Input: part model. Units: mm. Frame: model coordinates. Face numbers are marked on the shaded views. A direction names the side the tool comes from. Coordinates: 2 decimals unless noted, no trailing zeros. Order: outer loops, then holes, each group sorted by start corner. A loop starts at its lowest first (then second) coordinate and runs counter-clockwise, first axis right, second up. Notation, with made-up numbers: (59, 83.5) -> (90, 83.5) arc R14 ccw to (90, 109.5) -> close; hole circle Ø9 at (7, 33.5). An arc over 180 degrees is marked (long way). One line per item, written item: value. Start each with the question number.
from build123d import *

# Parameters (mm, degrees)
F1_DEPTH = 50.8
F3_DEPTH = 25.4
F4_DEPTH = 50.8


with BuildPart() as f1:
    # F0 (on Top) → F1 (new body)
    with BuildSketch(Plane.XY):
        with BuildLine():
            ThreePointArc((-15.1947466657, 0), (-22.0060110943, -10.86221038), (-25.7512666285, -23.1241025031))
            ThreePointArc((-25.7512666285, -23.1241025031), (-2.0484127491, -44.6133454073), (23.3222842216, -25.1212809235))
            ThreePointArc((23.3222842216, -25.1212809235), (21.5555211936, -11.7044416716), (14.7629464045, 0))
            ThreePointArc((14.7629464045, 0), (10.7387450248, 12.5467581674), (14.7629464045, 25.0935163349))
            ThreePointArc((14.7629464045, 25.0935163349), (21.5180813897, 36.4983696165), (23.3222842216, 49.63029176))
            Line((23.3222842216, 49.63029176), (-25.7512666285, 49.63029176))
            ThreePointArc((-25.7512666285, 49.63029176), (-22.2790381522, 36.5848904706), (-15.1947466657, 25.0935163349))
            ThreePointArc((-15.1947466657, 25.0935163349), (-10.9623069939, 12.5467581674), (-15.1947466657, 0))
        make_face()
    extrude(amount=F1_DEPTH)

    # F2 (on Right) → F3 (cut)
    with BuildSketch(Plane.YZ):
        with BuildLine():
            ThreePointArc((24.7435215861, 0), (0.6627701223, 5.5987162901), (-23.4179813415, 0))
            Line((-23.4179813415, 0), (24.7435215861, 0))
        make_face()
        with BuildLine():
            ThreePointArc((-46.2089851499, 24.0807514638), (-34.8134832457, 29.0446018263), (-23.4179813415, 24.0807514638))
            ThreePointArc((-23.4179813415, 24.0807514638), (0.6627701223, 14.6606816853), (24.7435215861, 24.0807514638))
            add(Edge.make_bspline(
                [(24.7435215861, 24.0807514638), (26.9770560839, 27.0474434767), (31.7641691677, 33.4059260361), (45.7356507893, 42.0064080333), (49.0760807653, 41.9577828011), (50.1966327429, 41.9414713979)],
                knots=[0, 0, 0, 0, 0.3675927898, 0.7878581036, 1, 1, 1, 1], degree=3))
            Line((50.1966327429, 41.9414713979), (50.1966327429, 52.80091241))
            Line((50.1966327429, 52.80091241), (-46.2089851499, 52.80091241))
            Line((-46.2089851499, 52.80091241), (-46.2089851499, 24.0807514638))
        make_face()
    extrude(amount=F3_DEPTH, mode=Mode.SUBTRACT)

    # F2 (on Right) → F4 (cut)
    with BuildSketch(Plane.YZ):
        with BuildLine():
            ThreePointArc((-46.2089851499, 24.0807514638), (-34.8134832457, 29.0446018263), (-23.4179813415, 24.0807514638))
            ThreePointArc((-23.4179813415, 24.0807514638), (0.6627701223, 14.6606816853), (24.7435215861, 24.0807514638))
            add(Edge.make_bspline(
                [(24.7435215861, 24.0807514638), (26.9770560839, 27.0474434767), (31.7641691677, 33.4059260361), (45.7356507893, 42.0064080333), (49.0760807653, 41.9577828011), (50.1966327429, 41.9414713979)],
                knots=[0, 0, 0, 0, 0.3675927898, 0.7878581036, 1, 1, 1, 1], degree=3))
            Line((50.1966327429, 41.9414713979), (50.1966327429, 52.80091241))
            Line((50.1966327429, 52.80091241), (-46.2089851499, 52.80091241))
            Line((-46.2089851499, 52.80091241), (-46.2089851499, 24.0807514638))
        make_face()
        with BuildLine():
            ThreePointArc((24.7435215861, 0), (0.6627701223, 5.5987162901), (-23.4179813415, 0))
            Line((-23.4179813415, 0), (24.7435215861, 0))
        make_face()
    extrude(amount=-F4_DEPTH, mode=Mode.SUBTRACT)


solid = f1.part
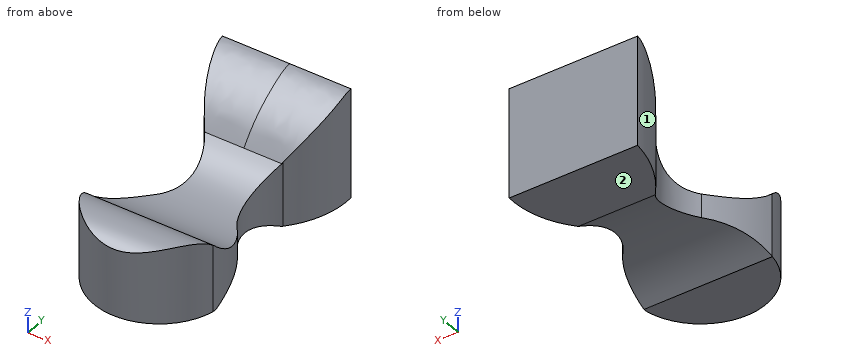
1) Section query A-A, the plane z = 9. Return the cut outline in (x, y), plus the area to 3 significant figures.
2) Ray query, line 1 along Y through (x, z) = (-16, 26); line 2 along Y through (x, z) = (17.5, 22); line 3 along X through (y, z) = (11, 8). Return the intervals inside material, ascending. Write a range as from..to.
3) Pin query (flat end, axial travel): pin 1 Ø8 at (x, y) = (11, 3) entering from +Z; pin 2 Ø12 at (y, z) = (-14, 18) entering from -X; pin 3 Ø10 at (y, z) = (-12, 7) entering from +X. Return the tip coordinate at first contact, or that it passes through.
4) Section query B-B, the plane y = 2. Return the cut outline in (x, z), plus the area to 3 significant figures.
5) Access query for the marked faces 1 and 2. Directions: +Z, -Z, +X, -X, +Y, -Y. A direction counts if a zero-diameter tool reaches every point of the face in a straight line with its end or side. Return the directions, or none.
6) Section query C-C, the plane y = -29. Return the cut outline in (x, z), plus the area to 3 significant figures.
Entries:
1. outline: (-25.75, -23.12) arc R24.96 ccw to (23.32, -25.12) arc R34.49 ccw to (14.76, 0) arc R21.57 cw to (14.76, 25.09) arc R33.51 ccw to (23.32, 49.63) -> (-25.75, 49.63) arc R46.35 ccw to (-15.19, 25.09) arc R20.71 cw to (-15.19, 0) arc R48.77 ccw to start
1. area: 3,450 mm2
2. line 1: y = -39.65..-25.57, 26.2..49.63
2. line 2: y = -36.39..-20.95, 28.56..49.63
2. line 3: x = -11.02..10.79
3. pin 1: stops at z = 15.23
3. pin 2: stops at x = -25.13
3. pin 3: stops at x = 22.9
4. outline: (-13.85, 5.58) -> (13.49, 5.58) -> (13.49, 14.69) -> (-13.85, 14.69) -> close
4. area: 249 mm2
5. face 1: +Z, -Z, -X
5. face 2: -Z, +X, -X, +Y, -Y
6. outline: (-24.18, 0) -> (22.12, 0) -> (22.12, 27.92) -> (-24.18, 27.92) -> close
6. area: 1,290 mm2
